Could you check a few things on this model? Use its own coordinates, in mm. A direction names the side the tool comes from. Round coordinates to 2 decimals unless told otherwise and drop trailing zeros. Write each loop counter-clockwise with the first axis right and the second up, starting at its lowest first coordinate (ties: lowest second). Pieces come first, ordered by that corner, then holes. Notation, with made-up numbers: (55.5, 78) -> (65.5, 78) arc R26 cw to (65.5, 106) -> close; hole circle Ø2 at (41.5, 82.5). An arc over 180 degrees is marked (long way). Answer as CSV lines item,"result". Start each with the question number.
Q1. If we mould it in two halves opening along Y, with no side actions, what happens to faces 5 (the flat face through (7.826, 16.725, 13.552)), 6 (the cylindrical face through (11.57, 26.03, -11.96)), 7 (the flat face through (3.522, 20.611, -63.226)), 8 (the cylindrical face through (7.826, 22.985, 0.517))? For each: pulls with the +Y half, pulls with the -Y half, needs draft (parallel to the pull), parting line crosses it, or undercut.
Q2. Will these pins go through, and if not, where does the flat tip stop? pin 1 Ø12.5 at (y, z) = (19.05, 0) entering from +X (3 decimals); pin 2 Ø5 at (x, z) = (4.5, -3) entering from -Y; pin 3 Ø5 at (x, y) = (2, 24.5) entering from +Z; pin 4 Ø3 at (x, z) = (6, -36) entering from +Y.
Q3. Imagine slicing it at B-B on x = 14.25. Please give me the cut outline in (y, z), and give its area (3 significant figures).
Q4. If I drill on line 1 (Y direction, x = 3.5, z = 0); line 2 (X direction, y = 24, z = -49.5); line 3 (Z direction, x = 9.25, y = 22), over which ranges is the centre line in solid material (lowest first)? Write a range as [from, to].
Q5. For faces 1 (the cylindrical face through (11.45, 35.63, -45.35)), 2 (the flat face through (4.3, 26.49, -43.58)), 3 (the flat face through (11.57, 31.723, -43.979)), 4 (the cylindrical face through (11.448, 28.635, -41.314)), which set-ups out of +Z, -Z, +X, -X, +Y, -Y let a thin tool reach every point of the face, with its end or its side?
Q6. Imagine slicing it at A-A on z = 0. Please give me the cut outline in (x, y) (3 decimals).
Q7. Imagine slicing it at C-C on z = -60. Please give me the cut outline in (x, y), and give its area (3 significant figures).
from build123d import *

# Parameters (mm, degrees)
SKETCH1_R           = 3.96875
BOSS_EXTRUDE1_DEPTH = 15.875
SKETCH2_R           = 3.175
SKETCH2_R_2         = 3.81
CUT_EXTRUDE1_DEPTH  = 9.525
CUT_EXTRUDE2_DEPTH  = 8.73125
FILLET1_R           = 2.54


with BuildPart() as part:
    # Sketch1 → Boss-Extrude1 (new body)
    with BuildSketch(Plane(origin=(0, 0, 0), x_dir=(0, 0, -1), z_dir=(1, 0, 0))):
        with BuildLine():
            ThreePointArc((-2.230020797, 12.263235579), (-6.186668978, 15.478125), (-6.992520797, 20.51212755))
            Line((-6.992520797, 20.51212755), (-16.129403285, 15.236945986))
            Line((-16.129403285, 15.236945986), (-11.366903285, 6.988054014))
            Line((-11.366903285, 6.988054014), (-2.230020797, 12.263235579))
        make_face()
        with BuildLine():
            Line((-6.992520797, 20.51212755), (2.230020797, 25.836764421))
            ThreePointArc((2.230020797, 25.836764421), (-3.571875, 25.236668978), (-6.992520797, 20.51212755))
        make_face()
        with BuildLine():
            Line((6.992520797, 17.58787245), (-2.230020797, 12.263235579))
            ThreePointArc((-2.230020797, 12.263235579), (3.571875, 12.863331022), (6.992520797, 17.58787245))
        make_face()
        with BuildLine():
            Line((65.622755111, 24.761945986), (32.995567884, 43.599261314))
            Line((32.995567884, 43.599261314), (2.230020797, 25.836764421))
            ThreePointArc((2.230020797, 25.836764421), (5.786357884, 23.239418396), (7.14375, 19.05))
            ThreePointArc((7.14375, 19.05), (7.105842121, 18.315036184), (6.992520797, 17.58787245))
            Line((6.992520797, 17.58787245), (32.995567884, 32.600738686))
            Line((32.995567884, 32.600738686), (60.860255111, 16.513054014))
            Line((60.860255111, 16.513054014), (65.622755111, 24.761945986))
        make_face()
        with BuildLine():
            ThreePointArc((7.14375, 19.05), (5.786357884, 23.239418396), (2.230020797, 25.836764421))
            Line((2.230020797, 25.836764421), (-6.992520797, 20.51212755))
            ThreePointArc((-6.992520797, 20.51212755), (-6.186668978, 15.478125), (-2.230020797, 12.263235579))
            Line((-2.230020797, 12.263235579), (6.992520797, 17.58787245))
            ThreePointArc((6.992520797, 17.58787245), (7.105842121, 18.315036184), (7.14375, 19.05))
        make_face()
        with Locations((0, 19.05)):
            Circle(SKETCH1_R, mode=Mode.SUBTRACT)
    extrude(amount=BOSS_EXTRUDE1_DEPTH)

    # Sketch2 → Cut-Extrude1 (cut)
    with BuildSketch(Plane(origin=(0, 18.411945986, 10.630141971), x_dir=(1, 0, 0), z_dir=(0, 0.866025404, 0.5))):
        with Locations((7.9375, 0)):
            Circle(SKETCH2_R)
        with Locations((7.9375, 22.225)):
            Circle(SKETCH2_R_2)
    extrude(amount=-CUT_EXTRUDE1_DEPTH, mode=Mode.SUBTRACT)

    # Sketch3 → Cut-Extrude2 (cut)
    with BuildSketch(Plane(origin=(15.875, 0, 0), x_dir=(0, 0, -1), z_dir=(1, 0, 0))):
        Polygon((65.622755111, 24.761945986), (60.860255111, 16.513054014), (41.612840512, 27.625554014), (46.375340512, 35.874445986), align=None)
    extrude(amount=-CUT_EXTRUDE2_DEPTH, mode=Mode.SUBTRACT)

    # Fillet1
    fillet1_edges = [part.edges().sort_by_distance(p)[0] for p in [
        (7.9375, 6.988054014, 11.366903285),
        (7.9375, 15.236945986, 16.129403285),
        (7.9375, 20.51212755, 6.992520797),
        (7.9375, 25.836764421, -2.230020797),
        (7.9375, 43.599261314, -32.995567884),
        (7.9375, 32.600738686, -32.995567884),
        (7.9375, 17.58787245, -6.992520797),
        (7.9375, 12.263235579, 2.230020797),
        (3.571875, 24.761945986, -65.622755111),
        (3.571875, 16.513054014, -60.860255111),
        (11.509375, 35.874445986, -46.375340512),
        (11.509375, 27.625554014, -41.612840512),
    ]]
    fillet(fillet1_edges, radius=FILLET1_R)


solid = part.part
Checks:
1,face 5,"pulls with the +Y half"
1,face 6,"undercut"
1,face 7,"pulls with the -Y half"
1,face 8,"undercut"
2,pin 1,"x = 15.875"
2,pin 2,"y = 11.92"
2,pin 3,"z = 6.51"
2,pin 4,"y = 42.73"
3,outline,"(8.26, 9.17) -> (11.75, 3.13) arc R2.54 cw to (12.04, 1.37) arc R7.14 ccw to (16.73, -6.76) arc R2.54 cw to (18.11, -7.89) -> (31.87, -31.73) arc R2.54 cw to (31.87, -34.27) -> (28.9, -39.41) arc R2.54 ccw to (29.83, -42.88) -> (33.67, -45.11) arc R2.54 ccw to (37.14, -44.18) -> (42.87, -34.27) arc R2.54 ccw to (42.87, -31.73) -> (26.35, -3.13) arc R2.54 cw to (26.06, -1.37) arc R7.14 ccw to (21.37, 6.76) arc R2.54 cw to (19.99, 7.89) -> (16.51, 13.93) arc R2.54 ccw to (13.04, 14.86) -> (9.19, 12.64) arc R2.54 ccw to start; hole circle Ø7.94 at (19.05, 0)"
3,area,"616 mm^2"
4,line 1,"[11.91, 15.08], [23.02, 26.19]"
4,line 2,"[0, 7.14]"
4,line 3,"[-8.83, -2.65], [2.65, 6.51]"
5,face 1,"-Z, +X"
5,face 2,"+X, -X, -Y"
5,face 3,"-Z, +X, -Y"
5,face 4,"+X, -Y"
6,outline,"(0, 11.906) -> (15.875, 11.906) -> (15.875, 15.081) -> (0, 15.081) -> close; (0, 23.019) -> (15.875, 23.019) -> (15.875, 26.194) -> (0, 26.194) -> close"
7,outline,"(0, 17.44) -> (7.14, 17.44) -> (7.14, 28.01) -> (0, 28.01) -> close"
7,area,"75.5 mm^2"
